Could you check a few things on this model? Use its own coordinates, in mm. A direction names the side the tool comes from. Round coordinates to 2 decimals unless told otherwise and drop trailing zeros. Order: outer loops, then holes, each group sorted by start corner. A loop starts at its lowest first (then second) coordinate and runs counter-clockwise, first axis right, second up. Notation, with made-up numbers: (14, -9.5) - (39, -9.5) arc R22 cw to (39, 18.5) - close; hole circle Ø4 at (45, 87.25). An arc over 180 degrees is marked (long way). Return JSON: item names as keys, results as strings. Group by question number.
from build123d import *

# Parameters (mm, degrees)
BOSS_EXTRUDE1_DEPTH = 1.524
FILLET1_R           = 0.254


with BuildPart() as part:
    # Sketch1 → Boss-Extrude1 (new body)
    with BuildSketch(Plane.XY):
        Polygon((-6.2865, -0.762), (-6.2865, -1.524), (-4.433524529, -1.524), (-4.433524529, -5.163998713), (-10.537505967, -3.903634867), (-10.84568392, -5.39615031), (-13.830714807, -4.779794404), (-13.522536854, -3.287278961), (-22.062151888, -1.524), (-11.049, -1.524), (-11.049, -0.762), align=None)
    extrude(amount=BOSS_EXTRUDE1_DEPTH)

    # Fillet1
    fillet1_edges = [part.edges().sort_by_distance(p)[0] for p in [
        (-22.062151888, -1.524, 0.762),
    ]]
    fillet(fillet1_edges, radius=FILLET1_R)


solid = part.part
1) Will these pins go through, and if not, where does the flat tip stop? pin 1 (0.5 mm diameter, centred on x = -5.5, z = 1, fed in from +Y); pin 2 (0.6 mm diameter, centred on y = -1.5, z = 0.5, fed in from -X).
2) I want a section at D-D, the plane y = -5. List the corners of the cut face in (x, z) for me.
3) For faces 5 (the flat face through (-13.68, -4.04, 0.75)), 6 (the flat face through (-10.69, -4.64, 0.75)), 7 (the flat face through (-5, -1.524, 1)), which set-ups out of +Z, -Z, +X, -X, +Y, -Y let a thin tool reach every point of the face, with its end or its side?
4) I want a section at A-A, the plane y = -4.05. List the corners of the cut face in (x, z) for me, plus the area to 3 significant figures.
5) I want a section at B-B, the plane z = 0.6. List the corners of the cut face in (x, y) for me.
6) If I drill on line 1 along X through (y, z) = (-1.3, 1.4); line 2 along Y through (x, z) = (-16.5, 1.2); line 3 along X through (y, z) = (-3.5, 1), over which ranges is the centre line in solid material (lowest first)? Write a range as from..to.
7) I want a section at C-C, the plane x = -16.75. List the corners of the cut face in (y, z) for me, plus the area to 3 significant figures.
8) We'd pull the mould along X, two halves only. Please class faces 1 (the flat face through (-7.443, -4.543, 0.751)), 2 (the flat face through (-12.32, -5.09, 0.75)), 3 (the flat face through (-10, -3, 1.524)), 4 (the flat face through (-4.434, -3, 1)): +X half, -X half, draft (parallel to the pull), parting line (faces both ways), or undercut.
Outcome:
{
 "1": {"pin 1": "y = -1.52", "pin 2": "x = -19.83"},
 "2": {"outline": "(-12.76, 0) - (-10.76, 0) - (-10.76, 1.52) - (-12.76, 1.52) - close; (-5.23, 0) - (-4.43, 0) - (-4.43, 1.52) - (-5.23, 1.52) - close"},
 "3": {"face 5": "+Z, -Z, -X", "face 6": "+Z, -Z, -Y", "face 7": "+Z, -Z, +X, +Y"},
 "4": {"outline": "(-13.68, 0) - (-10.57, 0) - (-10.57, 1.52) - (-13.68, 1.52) - close; (-9.83, 0) - (-4.43, 0) - (-4.43, 1.52) - (-9.83, 1.52) - close", "area": "13.0 mm^2"},
 "5": {"outline": "(-19.63, -2.03) - (-13.52, -3.29) - (-13.83, -4.78) - (-10.85, -5.4) - (-10.54, -3.9) - (-4.43, -5.16) - (-4.43, -1.52) - (-6.29, -1.52) - (-6.29, -0.76) - (-11.05, -0.76) - (-11.05, -1.52) - (-19.58, -1.52) arc R0.25 ccw to start"},
 "6": {"line 1": "-11.05..-6.29", "line 2": "-2.67..-1.52", "line 3": "-13.57..-4.43"},
 "7": {"outline": "(-2.62, 0) - (-1.52, 0) - (-1.52, 1.52) - (-2.62, 1.52) - close", "area": "1.67 mm^2"},
 "8": {"face 1": "undercut", "face 2": "-X half", "face 3": "draft", "face 4": "+X half"}
}
